```python
from build123d import *

# Parameters (mm, degrees)
F0_R     = 3.5
F1_DEPTH = 32.893
F3_DEPTH = 44.5826506487
F5_DEPTH = 32.894


# Not quite as in the source:
# - a feature names something its author has since deleted; it is built from what else it names


with BuildPart() as f1:
    # F0 (on Top) → F1 (new body)
    with BuildSketch(Plane.XY):
        with BuildLine():
            Line((-293, -19), (-293, 0))
            Line((-293, 0), (-394.6, 0))
            Line((-394.6, 0), (-394.6, -0.3249169361))
            ThreePointArc((-394.6, -0.3249169361), (-389.9738981677, -11.4236067086), (-378.9287209511, -16.1760579795))
            ThreePointArc((-378.9287209511, -16.1760579795), (-371.1660381492, -27.7809948386), (-374.8890577817, -41.2373289829))
            Line((-374.8890577817, -41.2373289829), (-278.3200451143, -19.2755622931))
            Line((-278.3200451143, -19.2755622931), (-293, -19))
        make_face()
        with Locations((-361.0937758916, -22.86)):
            Circle(F0_R, mode=Mode.SUBTRACT)
        with Locations((-327.5875517832, -15.24)):
            Circle(F0_R, mode=Mode.SUBTRACT)
    extrude(amount=-F1_DEPTH)

    # F2 (on face) → F3 (cut, through all)
    with BuildSketch(Plane(origin=(-9.5187600933, 41.855342378, 0), x_dir=(0.9751017202, 0.2217580556, 0), z_dir=(0.2217580556, -0.9751017202, 0))):
        Polygon((-275.6648659783, -32.893), (-275.6648659783, -14), (-374.6996750289, -32.893), align=None)
        Polygon((-374.6996750289, -18.8976), (-287.8981553787, -2.3343288283), (-275.6648659783, -14), (-275.6648659783, 0), (-374.6996750289, 0), align=None)
    extrude(amount=-F3_DEPTH, mode=Mode.SUBTRACT)

    # F4: F1 across plane


with BuildPart() as f1_1:
    add(f1.part)
    add(f1.part.mirror(Plane.XZ))

    # F5 (cut, through all): a face of the model
    f5_faces = [f1_1.faces().sort_by_distance(p)[0] for p in [
        (-387.4719249036, 0, 0),
    ]]
    extrude(f5_faces, amount=-F5_DEPTH, mode=Mode.SUBTRACT)


solid = f1_1.part
```
Input: part model. Units: mm. Frame: model coordinates. A direction names the side the tool comes from. Coordinates: 2 decimals unless noted, no trailing zeros. Loops run counter-clockwise (first coordinate to the right, second up) from the corner with the lowest first, then second, coordinate; pieces in that order, holes last.
Q1. Set-up query: faces 5 (the flat face through (-327.28, 30.41, -17.4)), 6 (the flat face through (-285.95, -19.83, -6.79)), 7 (the flat face through (-293, 0, -9)). Return all of +Z, -Z, +X, -X, +Y, -Y with unobstructed straight access to the full face (end or side cutting, diameter ignored); none if empty.
Results are:
face 5: +Z, -Z, +X, +Y
face 6: +Z, +X
face 7: +Z, -Z, +X
Q2. Line query: line 1 along Z through (x, y) = (-349, 28); line 2 along Y through (x, z) = (-320, -13); line 3 along Z through (x, y) = (-338, -27). Output: solid intervals per line, ascending.
Results are:
line 1: z = -27.52 to -13.52
line 2: y = -28.75 to 28.75
line 3: z = -25.43 to -11.43
Q3. Mould query, pull axis X, two halves, no side actions, for faces 1 (the cylindrical face through (-371.2, -27.58, -25.07)), 2 (the cylindrical face through (-357.755, 21.809, -22.455)), 3 (the cylindrical face through (-357.755, -21.809, -22.455)), 4 (the flat face through (-293.542, -3.73, -3.133)). Classes: +X half, -X half, draft (parallel to the pull), parting line (faces both ways), or undercut.
Results are:
face 1: -X half
face 2: undercut
face 3: undercut
face 4: +X half
Q4. Section B-B, the plane z = -12. Return the cut outline in (x, y), and give its area (3 significant figures).
Results are:
outline: (-347.2, 0) - (-339.64, -33.22) - (-280.37, -19.74) - (-280.48, -19.24) - (-293, -19) - (-293, 19) - (-280.48, 19.24) - (-280.37, 19.74) - (-339.64, 33.22) - close; hole circle Ø7 at (-327.59, -15.24); hole circle Ø7 at (-327.59, 15.24)
area: 2,830 mm2
Q5. Section D-D, the plane x = -341.5. Return the cut outline in (y, z).
Results are:
outline: (-33.64, -26.36) - (0, -24.94) - (33.64, -26.36) - (33.64, -12.36) - (0, -10.94) - (-33.64, -12.36) - close
Q6. Section C-C, the plane x = -288. Return the cut outline in (y, z).
Results are:
outline: (-21.48, -15.89) - (-19.09, -15.79) - (-19.09, -5.04) - (-21.48, -4.53) - close; (19.09, -15.79) - (21.48, -15.89) - (21.48, -4.53) - (19.09, -5.04) - close
Q7. Contact query for flat-ended pins moving along their axis: pin 1 (1.5 mm diameter, centred on y = -9, z = -8, fed in from +X); pin 2 (1.5 mm diameter, centred on x = -298.5, y = 23, fed in from +Z); pin 3 (12 mm diameter, centred on x = -328, z = -27.5, fed in from -Y). Output: stop coordinate, or through.
Results are:
pin 1: stops at x = -293
pin 2: stops at z = -3.77
pin 3: stops at y = -31.79
Q8. Section A-A, the plane y = -17.5. Return the cut outline in (x, z), and give its area (3 significant figures).
Results are:
outline: (-377.07, -32.29) - (-330.26, -23.59) - (-330.26, -9.59) - (-377.07, -18.3) - close; (-324.92, -22.59) - (-293, -16.66) - (-293, -2.66) - (-324.92, -8.59) - close
area: 1,100 mm2
